from build123d import *

# Parameters (mm, degrees)
SKETCH1_R             = 47.5
SKETCH1_R_2           = 32.5
BOSS_EXTRUDE1_DEPTH   = 6.5
SKETCH2_R             = 5
CUT_EXTRUDE1_DEPTH    = 68.488887974
M5X0_8_TAPPED_HOLE1_D = 4.2
FILLET1_R             = 0.5


with BuildPart() as part:
    # Sketch1 → Boss-Extrude1 (new body)
    with BuildSketch(Plane.XY):
        with Locations(Location((0, 0, 0), (0, 0, 180))):
            Circle(SKETCH1_R)
        with Locations(Location((0, 0, 0), (0, 0, 180))):
            Circle(SKETCH1_R_2, mode=Mode.SUBTRACT)
    extrude(amount=BOSS_EXTRUDE1_DEPTH)

    # Sketch2 → Cut-Extrude1 (cut, through all)
    with BuildSketch(Plane.XY):
        with Locations(Location((9.835123714, 36.705181399, 0), (0, 0, 180))):
            Circle(SKETCH2_R)
        with Locations(Location((26.870057685, 26.870057685, 0), (0, 0, 180))):
            Circle(SKETCH2_R)
        with Locations(Location((36.705181399, 9.835123714, 0), (0, 0, 180))):
            Circle(SKETCH2_R)
        with Locations(Location((36.705181399, -9.835123714, 0), (0, 0, 180))):
            Circle(SKETCH2_R)
        with Locations(Location((26.870057685, -26.870057685, 0), (0, 0, 180))):
            Circle(SKETCH2_R)
        with Locations(Location((9.835123714, -36.705181399, 0), (0, 0, 180))):
            Circle(SKETCH2_R)
        with Locations(Location((-9.835123714, -36.705181399, 0), (0, 0, 180))):
            Circle(SKETCH2_R)
        with Locations(Location((-26.870057685, -26.870057685, 0), (0, 0, 180))):
            Circle(SKETCH2_R)
        with Locations(Location((-36.705181399, -9.835123714, 0), (0, 0, 180))):
            Circle(SKETCH2_R)
        with Locations(Location((-36.705181399, 9.835123714, 0), (0, 0, 180))):
            Circle(SKETCH2_R)
        with Locations(Location((-26.870057685, 26.870057685, 0), (0, 0, 180))):
            Circle(SKETCH2_R)
        with Locations(Location((-9.835123714, 36.705181399, 0), (0, 0, 180))):
            Circle(SKETCH2_R)
    extrude(amount=CUT_EXTRUDE1_DEPTH, mode=Mode.SUBTRACT)

    # M5x0.8 Tapped Hole1 (through all)
    with Locations(Plane.XY.offset(6.5)):
        with Locations((0, 37.5), (-37.5, 0), (37.5, 0), (0, -37.5)):
            Hole(M5X0_8_TAPPED_HOLE1_D / 2)

    # Fillet1
    fillet1_edges = [part.edges().sort_by_distance(p)[0] for p in [
        (47.5, 0, 0),
        (47.5, 0, 6.5),
    ]]
    fillet(fillet1_edges, radius=FILLET1_R)


solid = part.part
Can you work these out from the model? Positions are in its coordinate system, mm. Give positions to 0.01 mm unless a question says otherwise; leave off trailing zeros. Write each loop counter-clockwise with the first axis right and the second up, starting at its lowest first coordinate (ties: lowest second). Pieces come first, ordered by that corner, then holes. Notation, with made-up numbers: (47.5, 44.5) -> (54.5, 44.5) arc R19 ccw to (54.5, 50.5) -> close; hole circle Ø4 at (-8.5, 69). An arc over 180 degrees is marked (long way). Answer as a JSON object with one key per item and string values. Group by question number.
Item 1: Suppose I cut it at A-A (x = 0). Please give me the cut outline in (y, z).
Item 2: Suppose I cut it at C-C (z = 4). State how many separate pieces and enclosed holes the cut face has, plus the area to 3 significant figures.
Item 3: Please list where these lines run through material, in increasing order: line 1 (Y direction, x = -25.5, z = 2); line 2 (Y direction, x = 7, z = 5.5); line 3 (X direction, y = 26.5, z = 5). Write a range as [from, to].
Item 4: We'd pull the mould along X, two halves only. Please class faces 1 (the face through (10.919, -31.824, 3.204)), 2 (the face through (10.3, 46.37, 3.21)), 3 (the face through (28, -18, 6.5)): +X half, -X half, draft (parallel to the pull), parting line (faces both ways), or undercut.
Item 5: I'm going to push flat-ended pins straight in: P1, Ø3, axis at y = -32.5, z = 4.5, coming from the -X side; P2, Ø3, axis at x = -19.5, z = 3, coming from the -Y side; P3, Ø1.5, axis at x = 35, z = 5, coming from the +Y side. Where does each tip first touch, or does it pass through?
Findings:
{
 "1": {"outline": "(-47.5, 0.5) arc R0.5 ccw to (-47, 0) -> (-39.6, 0) -> (-39.6, 6.5) -> (-47, 6.5) arc R0.5 ccw to (-47.5, 6) -> close; (-35.4, 0) -> (-32.5, 0) -> (-32.5, 6.5) -> (-35.4, 6.5) -> close; (32.5, 0) -> (35.4, 0) -> (35.4, 6.5) -> (32.5, 6.5) -> close; (39.6, 0) -> (47, 0) arc R0.5 ccw to (47.5, 0.5) -> (47.5, 6) arc R0.5 ccw to (47, 6.5) -> (39.6, 6.5) -> close"},
 "2": {"separate pieces": "1", "enclosed holes": "17", "area": "2,770 mm²"},
 "3": {"line 1": "y = [-40.07, -31.68], [-22.06, -20.15], [20.15, 22.06], [31.68, 40.07]", "line 2": "y = [-46.98, -40.82], [-32.59, -31.74], [31.74, 32.59], [40.82, 46.98]", "line 3": "x = [-39.42, -31.86], [-21.88, -18.81], [18.81, 21.88], [31.86, 39.42]"},
 "4": {"face 1": "undercut", "face 2": "parting line", "face 3": "draft"},
 "5": {"P1": "stops at x = -35.99", "P2": "stops at y = -43.96", "P3": "stops at y = 32.91"}
}
